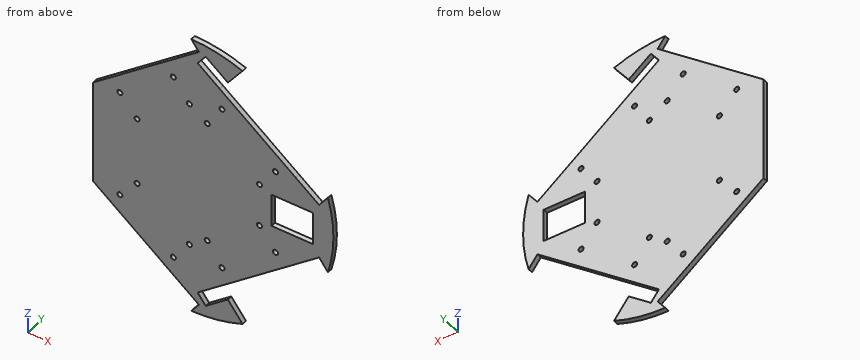
Autodesk Inventor part; units mm, degrees
ref_plane "YZ Plane" through (0, 0, 0) normal (1, 0, 0) x (0, 1, 0)
ref_plane "XZ Plane" through (0, 0, 0) normal (0, 1, 0) x (-1, 0, 0)
ref_plane "XY Plane" through (0, 0, 0) normal (0, 0, 1) x (1, 0, 0)
sketch "Boceto1" plane through (0, 0, 0) normal (0, 1, 0) x (-1, 0, 0)
  line L0 (0, 0) -> (0, -87) construction
  line L1 (0, 0) -> (0, 83.8978) construction
  line L2 (0, 0) -> (-87, 0) construction
  line L3 (0, 0) -> (59, 0) construction
  line L4 (-74.5, -10) -> (-49.5, -10)
  line L5 (-49.5, -10) -> (-49.5, 10)
  line L6 (-49.5, 10) -> (-74.5, 10)
  line L7 (-74.5, 10) -> (-74.5, -10)
  line L8 (-74.5, -10) -> (-49.5, 10) construction
  line L9 (-49.5, -10) -> (-74.5, 10) construction
  line L10 (-18, 63.0769) -> (-64.0145, 27.7688)
  line L11 (9, 69.9829) -> (55.0145, 34.6747)
  line L12 (9, 69.9829) -> (20.2282, 84.6157)
  line L13 (-18, 63.0769) -> (-31.752, 80.9988)
  line L14 (-64.0145, 27.7688) -> (-75.6609, 42.9467)
  line L15 (-18, -63.0769) -> (-64.0145, -27.7688)
  line L16 (9, -69.9829) -> (55.0145, -34.6747)
  line L17 (9, -69.9829) -> (20.2282, -84.6157)
  line L18 (-18, -63.0769) -> (-31.752, -80.9988)
  line L19 (-64.0145, -27.7688) -> (-75.6609, -42.9467)
  arc A0 (-75.6609, 42.9467) -> (-75.6609, -42.9467) centre (0, 0) ccw
  arc A1 (20.2282, 84.6157) -> (-31.752, 80.9988) centre (0, 0) ccw
  arc A2 (-31.752, -80.9988) -> (20.2282, -84.6157) centre (0, 0) ccw
  line L20 (59, 37.9189) -> (59, -37.9189)
  line L21 (58.0583, 38.6415) -> (59, 37.9189)
  line L22 (55.0145, 34.6747) -> (58.0583, 38.6415)
  line L23 (58.0583, -38.6415) -> (59, -37.9189)
  line L24 (55.0145, -34.6747) -> (58.0583, -38.6415)
  circle A3 centre (-19.2647, 50.7623) radius 1.55
  circle A4 centre (-51.7921, 25.8031) radius 1.55
  line L25 (-41.0072, 45.4229) -> (-35.5284, 38.2827) construction
  line L26 (-19.2647, 50.7623) -> (-51.7921, 25.8031) construction
  line L27 (32.0072, 52.3288) -> (22.9685, 40.5493) construction
  circle A5 centre (10.2647, 57.6682) radius 1.55
  circle A6 centre (42.7921, 32.709) radius 1.55
  circle A7 centre (-19.2647, -50.7623) radius 1.55
  circle A8 centre (-51.7921, -25.8031) radius 1.55
  circle A9 centre (10.2647, -57.6682) radius 1.55
  circle A10 centre (42.7921, -32.709) radius 1.55
  line L28 (42.7921, 32.709) -> (10.2647, 57.6682) construction
  point P0 (-62, 0)
  point P1 (-74.5, 0)
  point P2 (26.5284, 45.1886)
  dimension "d1" = 25
  dimension "d2" = 20
  dimension "d9" = 52.5
  dimension "d10" = 52.5
  dimension "d11" = 61
  dimension "d12" = 61
  dimension "d13" = 58
  dimension "d17" = 90
  dimension "d18" = 9
  dimension "d19" = 18
  dimension "d20" = 58
  dimension "d21" = 90
  dimension "d22" = 90
  dimension "d23" = 87
  dimension "d24" = 87
  dimension "d26" = 59
  dimension "d27" = 5
  dimension "d28" = 5
  dimension "d29" = 3.1
  dimension "d30" = 3.1
  dimension "d31" = 41
  dimension "d32" = 9
  dimension "d37" = 90
  dimension "d38" = 3.1
  dimension "d39" = 3.1
  dimension "d40" = 41
  dimension "d41" = 9
  dimension "d54" = 62
extrude "Extrusión1" add sketch "Boceto1" along normal blind 3
sketch "Boceto2" plane through (0, 3, 0) normal (0, 1, 0) x (1, 0, 0)
  line L0 (-9, -69.9829) -> (-55.0145, -34.6747)
  line L1 (-32.0072, -52.3288) -> (-0.1642, -10.8301) construction
  circle A0 centre (-32.2776, -20.6489) radius 1.55
  circle A1 centre (-0.5435, -44.9994) radius 1.55
  line L2 (-32.2776, -20.6489) -> (-0.5435, -44.9994) construction
  circle A2 centre (-42.7921, -32.709) radius 1.55 construction
  line L3 (64.0145, -27.7688) -> (18, -63.0769)
  line L4 (41.0072, -45.4229) -> (14.3892, -10.7335) construction
  circle A3 centre (10.3178, -37.4599) radius 1.55
  circle A4 centre (42.052, -13.1094) radius 1.55
  line L5 (42.052, -13.1094) -> (10.3178, -37.4599) construction
  circle A5 centre (19.2647, -50.7623) radius 1.55 construction
  line L6 (-59, 37.9189) -> (-59, -37.9189) construction
  line L7 (-59, 0) -> (115.874, 0) construction
  circle A6 centre (-32.2776, 20.6489) radius 1.55
  circle A7 centre (-0.5435, 44.9994) radius 1.55
  circle A8 centre (10.3178, 37.4599) radius 1.55
  circle A9 centre (42.052, 13.1094) radius 1.55
  point P0 (0, 0)
  dimension "d44" = 3.1
  dimension "d45" = 3.1
  dimension "d46" = 19.5
  dimension "d47" = 40
  dimension "d48" = 16
  dimension "d51" = 16
  dimension "d52" = 19.5
  dimension "d53" = 40
extrude "Extrusión2" cut sketch "Boceto2" against normal blind 10
sketch "Boceto3" plane through (0, 3, 0) normal (0, 1, 0) x (1, 0, 0)
  circle A0 centre (0, 0) radius 90 construction
  dimension "d55" = 180
sketch "Boceto5" plane through (0, 3, 0) normal (0, 1, 0) x (1, 0, 0)
  arc A0 (75.6609, 42.9467) -> (75.6609, -42.9467) centre (0, 0) ccw construction
  line L0 (87, 0) -> (-107.1861, 0) construction
  line L1 (-9, -69.9829) -> (-55.0145, -34.6747)
  line L2 (-9, -69.9829) -> (5.2804, -80.9406)
  line L3 (5.2804, -80.9406) -> (0.6326, -86.9977)
  arc A1 (31.752, -80.9988) -> (-20.2282, -84.6157) centre (0, 0) ccw
  line L4 (18, -63.0769) -> (31.752, -80.9988)
  line L5 (18, -63.0769) -> (4.513, -73.4259)
  line L6 (4.513, -73.4259) -> (9.3831, -79.7727)
  line L7 (9.3831, -79.7727) -> (22.8701, -69.4238)
  line L8 (-55.0145, -34.6747) -> (-59, -31.6165)
  line L9 (-59, -37.9189) -> (-59, 37.9189)
  circle A2 centre (42.052, 13.1094) radius 1.55
  circle A3 centre (-32.2776, -20.6489) radius 1.55
  circle A4 centre (-32.2776, 20.6489) radius 1.55
  circle A5 centre (42.052, -13.1094) radius 1.55
  circle A6 centre (10.3178, 37.4599) radius 1.55
  circle A7 centre (-0.5435, -44.9994) radius 1.55
  circle A8 centre (-0.5435, 44.9994) radius 1.55
  circle A9 centre (10.3178, -37.4599) radius 1.55
  arc A10 (-20.2282, -84.6157) -> (31.752, -80.9988) centre (0, 0) ccw
  line L10 (18, -63.0769) -> (31.752, -80.9988)
  line L11 (64.0145, -27.7688) -> (18, -63.0769)
  line L12 (75.6609, -42.9467) -> (64.0145, -27.7688)
  arc A11 (75.6609, -42.9467) -> (75.6609, 42.9467) centre (0, 0) ccw
  line L13 (64.0145, 27.7688) -> (75.6609, 42.9467)
  line L14 (18, 63.0769) -> (64.0145, 27.7688)
  line L15 (31.752, 80.9988) -> (18, 63.0769)
  arc A12 (31.752, 80.9988) -> (-20.2282, 84.6157) centre (0, 0) ccw
  line L16 (-9, 69.9829) -> (-20.2282, 84.6157)
  line L17 (-55.0145, 34.6747) -> (-9, 69.9829)
  line L18 (-58.0583, 38.6415) -> (-55.0145, 34.6747)
  line L19 (-59, 37.9189) -> (-58.0583, 38.6415)
  line L20 (-59, -37.9189) -> (-59, 37.9189)
  line L21 (-58.0583, -38.6415) -> (-59, -37.9189)
  line L22 (-55.0145, -34.6747) -> (-58.0583, -38.6415)
  line L23 (-9, -69.9829) -> (-55.0145, -34.6747)
  line L24 (-20.2282, -84.6157) -> (-9, -69.9829)
  circle A13 centre (-42.7921, 32.709) radius 1.55
  circle A14 centre (-10.2647, 57.6682) radius 1.55
  circle A15 centre (19.2647, 50.7623) radius 1.55
  circle A16 centre (51.7921, 25.8031) radius 1.55
  circle A17 centre (-42.7921, -32.709) radius 1.55
  circle A18 centre (-10.2647, -57.6682) radius 1.55
  circle A19 centre (51.7921, -25.8031) radius 1.55
  circle A20 centre (19.2647, -50.7623) radius 1.55
  line L25 (74.5, -10) -> (74.5, 10)
  line L26 (49.5, -10) -> (74.5, -10)
  line L27 (49.5, 10) -> (49.5, -10)
  line L28 (74.5, 10) -> (49.5, 10)
  line L29 (64.0145, -27.7688) -> (18, -63.0769)
  line L30 (64.0145, -27.7688) -> (78.2949, -16.8111)
  line L31 (78.2949, -16.8111) -> (83.6749, -23.8225)
  point P0 (-55.0145, -34.6747)
  point P1 (-9, -69.9829)
  point P2 (-20.2282, -84.6157)
  point P3 (-20.2282, 84.6157)
  point P4 (31.752, -80.9988)
  point P5 (75.6609, 42.9467)
  point P6 (-20.2282, -84.6157)
  dimension "d66" = 18
  dimension "d67" = 17
  dimension "d68" = 8
  dimension "d69" = 18
extrude "Extrusión3" cut sketch "Boceto5" against normal blind 10 contours L24 A1 L16 L17 L18 L19 L9 L21 L22 L1 | L2 L3 A10 L24 | L22 L21 L9 L8 | L4 L11 L12 A1 | A1 L13 L14 L15 | L12 L30 L31 A1 | L7 L6 L5 L4
mirror "Simetría1" about plane through (0, 0, 0) normal (0, 0, 1) of "Extrusión3"
ref_plane "Plano de trabajo1" through (0, 0, 0) normal (0, 0, 1) x (1, 0, 0)
properties part number "newbasecentral"
The model under review builds one solid part; all positions refer to its coordinate system, in mm. Round coordinates to 2 decimals unless told otherwise and drop trailing zeros. Write each loop counter-clockwise with the first axis right and the second up, starting at its lowest first coordinate (ties: lowest second). Pieces come first, ordered by that corner, then holes. Notation, with made-up numbers: M 35.5,-7.75 L 63.5,-7.75 A27 cw 63.5,17.25 Z; hole C 44.5,18.5 d2. An arc over 180 degrees is marked long. Use a Markdown table: item, result. Add a question column.
Q1. To check wall thickness, follow line 1 (Z direction, x = 24, y = 0.6); line 2 (X direction, y = 2.85, z = -0.5); line 3 (X direction, y = 1.55, z = 4). State the ranges of each line that lie inside material, in increasing order.
Q2. We need section A-A, the plane z = 3.5. State the section outline as (x, y) points.
Q3. We need section B-B, the plane x = 27. State the section outline as (y, z) points.
Q4. We need section D-D, the plane y = 1.75. Count the separate pieces of the cut face and the enclosed holes in it, plus the area to 3 significant figures.
Q5. We need section C-C, the plane x = 69.5. State the section outline as (y, z) points.
Q6. Insertion check: pin 1 (3 mm diameter, centred on x = 10.32, z = 37.46, fed in from -Y); pin 2 (1.5 mm diameter, centred on x = 23.5, y = 1, fed in from -Z). Each pin has a flat end and moves straight along its axis. Give the tip position at first contact, or say it passes through.
Findings below:
| question | item | result |
|---|---|---|
| 1 | line 1 | z = -83.62 to -70.9, -58.47 to 58.47, 70.9 to 83.62 |
| 1 | line 2 | x = -59 to 49.5, 74.5 to 87 |
| 1 | line 3 | x = -59 to 49.5, 74.5 to 86.91 |
| 2 | outline | M -59,0 L 49.5,0 L 49.5,3 L -59,3 Z; M 74.5,0 L 86.93,0 L 86.93,3 L 74.5,3 Z |
| 3 | outline | M 0,-82.7 L 3,-82.7 L 3,-74.81 L 0,-74.81 Z; M 0,-56.17 L 3,-56.17 L 3,56.17 L 0,56.17 Z; M 0,74.81 L 3,74.81 L 3,82.7 L 0,82.7 Z |
| 4 | separate pieces | 1 |
| 4 | enclosed holes | 17 |
| 4 | area | 14,000 mm² |
| 5 | outline | M 0,-23.56 L 3,-23.56 L 3,-10 L 0,-10 Z; M 0,10 L 3,10 L 3,23.56 L 0,23.56 Z |
| 6 | pin 1 | passes through |
| 6 | pin 2 | stops at z = -83.97 |
